Verification items for the finished model (mm, model axes). Round coordinates to 2 decimals unless told otherwise and drop trailing zeros. Write each loop counter-clockwise with the first axis right and the second up, starting at its lowest first coordinate (ties: lowest second). Pieces come first, ordered by that corner, then holes. Notation, with made-up numbers: M 22,26.25 L 42,26.25 A14 cw 42,50.25 Z; hole C 19.25,52.5 d5. An arc over 180 degrees is marked long. One line per question, with ' | ' between items.
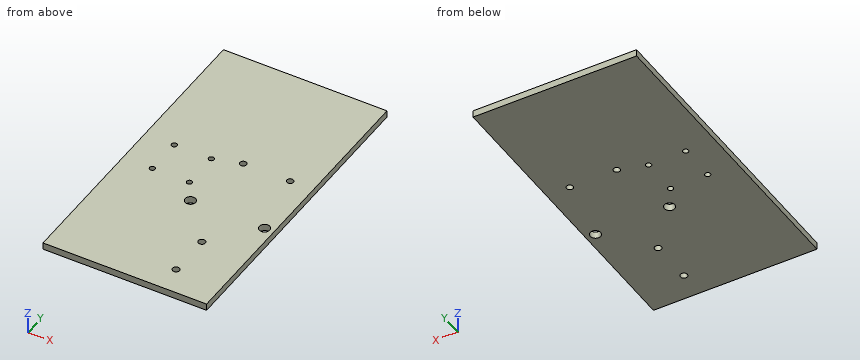
from build123d import *

# Parameters (mm, degrees)
SKETCH1_W           = 150
SKETCH1_H           = 280
BOSS_EXTRUDE1_DEPTH = 6.35
SKETCH4_R           = 3.175
SKETCH4_R_2         = 3
CUT_EXTRUDE1_DEPTH  = 6.35
CUT_EXTRUDE2_DEPTH  = 6.35


with BuildPart() as part:
    # Sketch1 → Boss-Extrude1 (new body)
    with BuildSketch(Plane.XY):
        with Locations((75, 140)):
            Rectangle(SKETCH1_W, SKETCH1_H)
    extrude(amount=BOSS_EXTRUDE1_DEPTH)

    # Sketch4 → Cut-Extrude1 (cut)
    with BuildSketch(Plane.XY):
        with Locations(Location((107.25, 25, 0), (0, 0, 180))):
            Circle(SKETCH4_R)
        with BuildLine():
            ThreePointArc((141.25, 109.597983852), (136.45, 104.797983852), (141.25, 99.997983852))
            ThreePointArc((141.25, 99.997983852), (146.05, 104.797983852), (141.25, 109.597983852))
        make_face()
        with BuildLine():
            ThreePointArc((73.25, 99.997983852), (78.05, 104.797983852), (73.25, 109.597983852))
            ThreePointArc((73.25, 109.597983852), (68.45, 104.797983852), (73.25, 99.997983852))
        make_face()
        with Locations(Location((128.750000003, 165.627983852, 0), (0, 0, 180))):
            Circle(SKETCH4_R_2)
        with Locations(Location((85.750000003, 165.627983852, 0), (0, 0, 180))):
            Circle(SKETCH4_R_2)
        with Locations(Location((107.25, 65, 0), (0, 0, 180))):
            Circle(SKETCH4_R)
    extrude(amount=CUT_EXTRUDE1_DEPTH, mode=Mode.SUBTRACT)

    # Sketch5 → Cut-Extrude2 (cut)
    with BuildSketch(Plane(origin=(0, 0, 6.35), x_dir=(-1, 0, 0), z_dir=(0, 0, 1))):
        with BuildLine():
            ThreePointArc((-61, -155.5), (-63.5, -158), (-61, -160.5))
            ThreePointArc((-61, -160.5), (-58.5, -158), (-61, -155.5))
        make_face()
        with BuildLine():
            ThreePointArc((-27, -155.5), (-29.5, -158), (-27, -160.5))
            ThreePointArc((-27, -160.5), (-24.5, -158), (-27, -155.5))
        make_face()
        with BuildLine():
            ThreePointArc((-27, -121.5), (-29.5, -124), (-27, -126.5))
            ThreePointArc((-27, -126.5), (-24.5, -124), (-27, -121.5))
        make_face()
        with BuildLine():
            ThreePointArc((-61, -126.5), (-58.5, -124), (-61, -121.5))
            ThreePointArc((-61, -121.5), (-63.5, -124), (-61, -126.5))
        make_face()
    extrude(amount=-CUT_EXTRUDE2_DEPTH, mode=Mode.SUBTRACT)


solid = part.part
1. Section check A-A, the plane y = 25. Record the cut outline in (x, z) (3 decimals), then the cut area to 3 significant figures.
Results:
outline: M 0,0 L 104.075,0 L 104.075,6.35 L 0,6.35 Z; M 110.425,0 L 150,0 L 150,6.35 L 110.425,6.35 Z | area: 912 mm2
2. Thickness scan on line 1 (X direction, y = 158, z = 3); line 2 (X direction, y = 165.5, z = 3.5); line 3 (Y direction, x = 72.5, z = 1.5). Record the ranges inside material, lowest first.
Results:
line 1: x = 0 to 24.5, 29.5 to 58.5, 63.5 to 150 | line 2: x = 0 to 82.75, 88.75 to 125.75, 131.75 to 150 | line 3: y = 0 to 100.06, 109.54 to 280
3. Section check B-B, the plane x = 128.75. Record the cut outline in (y, z), then the cut area to 3 significant figures.
Results:
outline: M 0,0 L 162.63,0 L 162.63,6.35 L 0,6.35 Z; M 168.63,0 L 280,0 L 280,6.35 L 168.63,6.35 Z | area: 1,740 mm2
